Verification items for the finished model (mm, model axes). Face numbers are marked on the shaded views. Give positions to 0.01 mm unless a question says otherwise; leave off trailing zeros. Write each loop counter-clockwise with the first axis right and the second up, starting at its lowest first coordinate (ties: lowest second). Pieces come first, ordered by that corner, then holes.
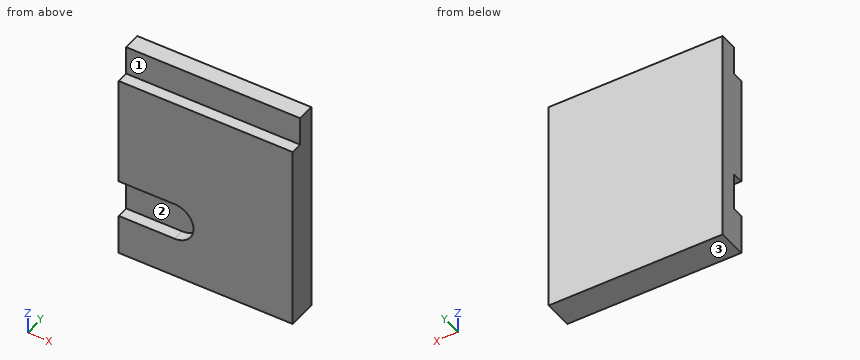
from build123d import *

# Parameters (mm, degrees)
F0_W     = 120
F0_H     = 20
F1_DEPTH = 12
F2_DEPTH = 20
F3_DEPTH = 20
F4_DEPTH = 20
F5_DEPTH = 12


with BuildPart() as f1:
    # F0 (on Front) → F1 (new body)
    with BuildSketch(Plane.XZ):
        with Locations((-60, 85.875011)):
            Rectangle(F0_W, F0_H)
    extrude(amount=F1_DEPTH)

    # F0 (on Front) → F2 (join)
    with BuildSketch(Plane.XZ):
        Polygon((0, 75.875011), (-120, 75.875011), (-120, 0), (-81.5, 0), (0, 0), align=None)
    extrude(amount=F2_DEPTH)

    # F0 (on Front) → F3 (join)
    with BuildSketch(Plane.XZ):
        with BuildLine():
            Line((0, 0), (-81.5, 0))
            ThreePointArc((-81.5, 0), (-68.437506, -13.062494), (-81.5, -26.124989))
            Line((-81.5, -26.124989), (0, -26.124989))
            Line((0, -26.124989), (0, -1.124989))
            Line((0, -1.124989), (0, 0))
        make_face()
    extrude(amount=F3_DEPTH)

    # F0 (on Front) → F4 (join)
    with BuildSketch(Plane.XZ):
        Polygon((-81.5, -26.124989), (-120, -26.124989), (-120, -54.124989), (0, -54.124989), (0, -26.124989), align=None)
    extrude(amount=F4_DEPTH)

    # F0 (on Front) → F5 (join)
    with BuildSketch(Plane.XZ):
        with BuildLine():
            Line((-81.5, 0), (-120, 0))
            Line((-120, 0), (-120, -26.124989))
            Line((-120, -26.124989), (-81.5, -26.124989))
            ThreePointArc((-81.5, -26.124989), (-68.437506, -13.062494), (-81.5, 0))
        make_face()
    extrude(amount=F5_DEPTH)


solid = f1.part
Item 1: Release check for a two-part mould opening along Z. For the marked faces 1, 2 and 3 record: released by +Z, released by -Z, zero draft, split by the parting line, or undercut.
Answer key:
face 1: zero draft
face 2: undercut
face 3: released by -Z
Item 2: Sectioned sample at C-C on x = -101. Record the cut outline in (y, z).
Answer key:
outline: (-20, -54.12) - (0, -54.12) - (0, 95.88) - (-12, 95.88) - (-12, 75.88) - (-20, 75.88) - (-20, 0) - (-12, 0) - (-12, -26.12) - (-20, -26.12) - close
Item 3: Sectioned sample at D-D on z = -13.5. Record the cut outline in (x, y).
Answer key:
outline: (-120, -12) - (-68.44, -12) - (-68.44, -20) - (0, -20) - (0, 0) - (-120, 0) - close
Item 4: Depth check by flat-ended pin: pin 1 (6 mm diameter, centred on x = -56, z = 89.5, fed in from -Y). Enter the tip coordinate at first touch or a pass-through.
Answer key:
pin 1: stops at y = -12
Item 5: Sectioned sample at B-B on y = -18.25. Record the cut outline in (x, z).
Answer key:
outline: (-120, -54.12) - (0, -54.12) - (0, 75.88) - (-120, 75.88) - (-120, 0) - (-81.5, 0) arc R13.06 cw to (-81.5, -26.12) - (-120, -26.12) - close
Item 6: Sectioned sample at A-A on x = -59.5. Record the cut outline in (y, z), then the cut area to 3 significant figures.
Answer key:
outline: (-20, -54.12) - (0, -54.12) - (0, 95.88) - (-12, 95.88) - (-12, 75.88) - (-20, 75.88) - close
area: 2,840 mm2
Item 7: Scan lines: line 1 along Z through (x, y) = (-42.5, -17.5); line 2 along Y through (x, z) = (-60, 84); line 3 along X through (y, z) = (-18.75, -23.5). Record each from-to range of solid material in increasing order.
Answer key:
line 1: z = -54.12 to 75.88
line 2: y = -12 to 0
line 3: x = -73.65 to 0
